Study the drawing (mm; zero at the part's minimum x, y, z) and answer. A direction names the side the tool comes from. Give positions to 0.01 mm unless a question says otherwise; leave off trailing zeros. Write each loop counter-clockwise with the first axis right and the second up, starting at its lowest first coordinate (ties: lowest second). Pieces come first, ordered by that corner, then holes. Notation, with made-up numbers: (-31, 33.25) - (-27, 33.25) arc R13 cw to (-27, 54.25) - close; hole circle Ø9 at (71, 58). An arc over 180 degrees is marked (long way). Write each question's results on one line, items separated by ' | '. Start each with the question number.
Q1. For the marked faces 1 and 2, determine the directions among +Z, -Z, +X, -X, +Y, -Y from which every point of the face is accessible in a straight line to the end or side of a thin tool.
Q2. Flat-ended cylindrical pins translate along their axes: pin 1 Ø4 at (y, z) = (8, 6) entering from -X; pin 2 Ø2.5 at (x, z) = (29, 4.5) entering from +Y; pin 3 Ø5 at (x, y) = (33, 8) entering from -Z; pin 4 Ø4 at (x, z) = (14, 2.5) entering from -Y. Find the tip coordinate at first contact, or state that the pin passes through.
Q3. Find the intervals of material crossed by probe 1 along X at (y, z) = (7.75, 3.25); probe 2 along Z at (x, y) = (22.5, 4.75); probe 3 along X at (y, z) = (8, 7), in increasing order.
Q4. Section C-C (x = 35) is taken. Determine the outline of the cut face in (y, z), plus the area to 3 significant figures.
Q5. Section B-B (y = 2.25) is taken. Determine the outline of the cut face in (x, z), plus the area to 3 significant figures.
Q6. Section A-A (z = 4.5) is taken. Determine the outline of the cut face in (x, y), plus the area to 3 significant figures.
Q7. Section D-D (x = 16) is taken. Determine the outline of the cut face in (y, z).
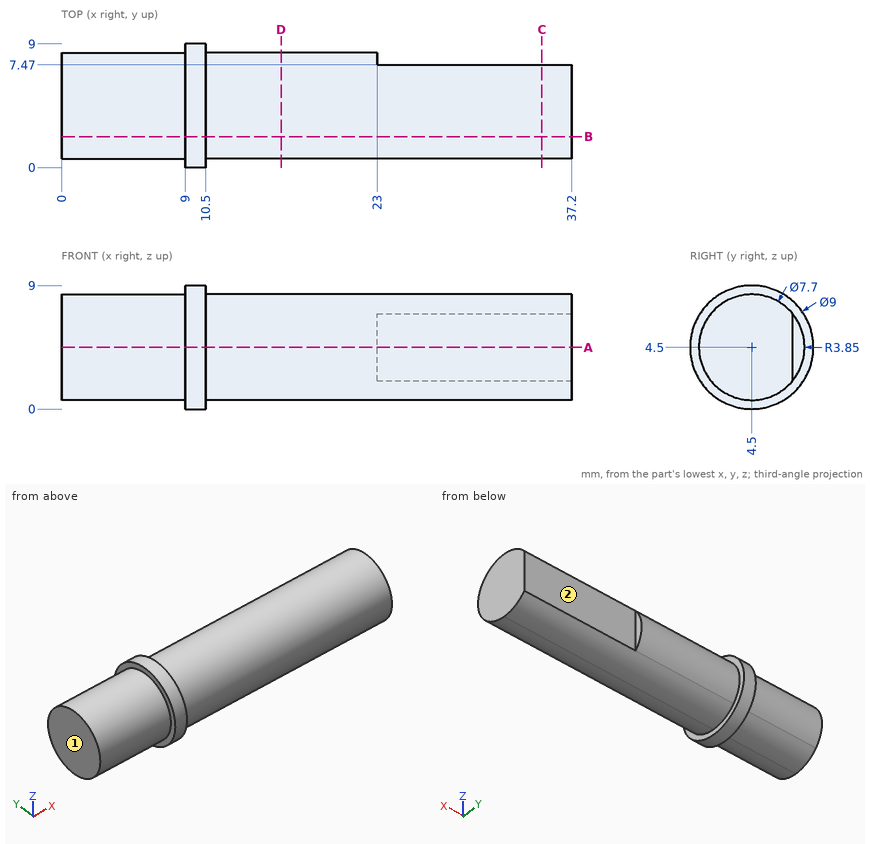
Answers below:
1) face 1: +Z, -Z, -X, +Y, -Y | face 2: +Z, -Z, +X, +Y
2) pin 1: stops at x = 0 | pin 2: stops at y = 7.47 | pin 3: stops at z = 0.78 | pin 4: stops at y = 0.65
3) probe 1: x = 0 to 23 | probe 2: z = 0.66 to 8.34 | probe 3: x = 9 to 10.5
4) outline: (7.47, 2.05) - (7.47, 6.95) arc R3.85 ccw (long way) to start | area: 43.6 mm2
5) outline: (0, 1.38) - (9, 1.38) - (9, 0.6) - (10.5, 0.6) - (10.5, 1.38) - (37.2, 1.38) - (37.2, 7.62) - (10.5, 7.62) - (10.5, 8.4) - (9, 8.4) - (9, 7.62) - (0, 7.62) - close | area: 235 mm2
6) outline: (0, 0.65) - (9, 0.65) - (9, 0) - (10.5, 0) - (10.5, 0.65) - (37.2, 0.65) - (37.2, 7.47) - (23, 7.47) - (23, 8.35) - (10.5, 8.35) - (10.5, 9) - (9, 9) - (9, 8.35) - (0, 8.35) - close | area: 276 mm2
7) outline: circle Ø7.7 at (4.5, 4.5)
